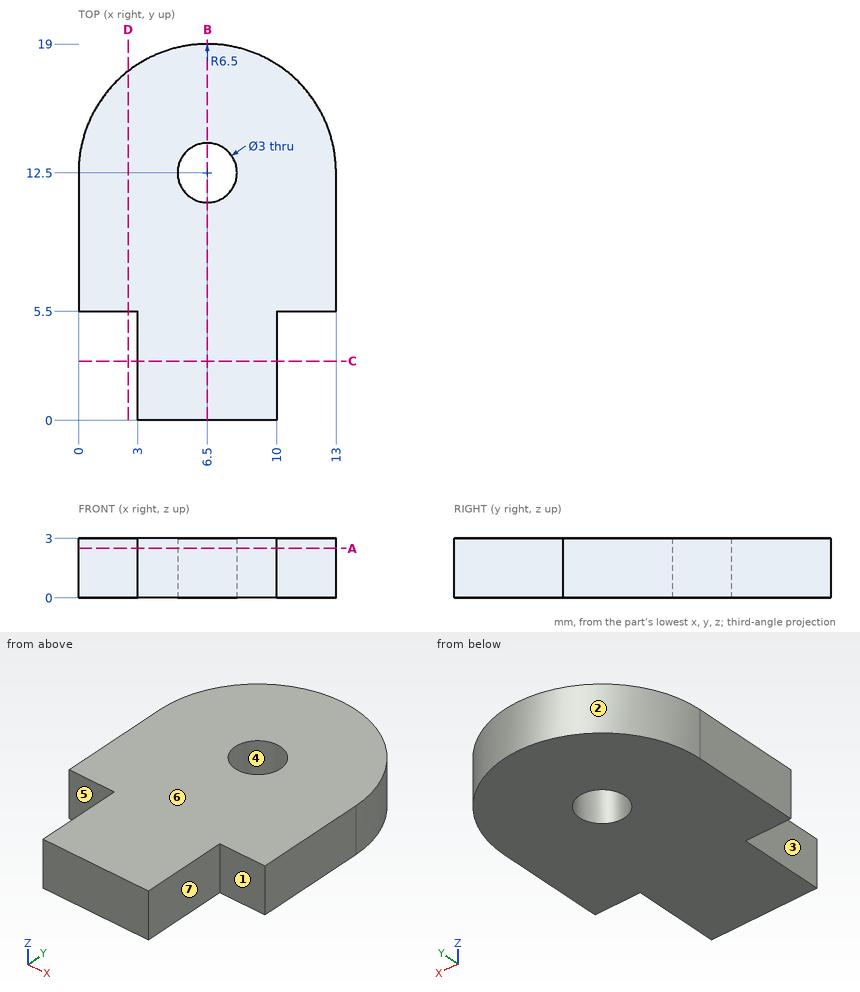
Check sheet for the drawn part. Datum: minimum x, y, z corner. Units: mm. A direction names the side the tool comes from. Round coordinates to 2 decimals unless told otherwise and drop trailing zeros. Loops run counter-clockwise (first coordinate to the right, second up) from the corner with the lowest first, then second, coordinate; pieces in that order, holes last. Notation, with made-up numbers: M 69.5,11 L 127.5,11 A37 ccw 127.5,49 Z; hole C -3.5,51.25 d10. An arc over 180 degrees is marked long. One line per question, with ' | ' between items. Start each with the question number.
Item 1: Release check for a two-part mould opening along Y. For the marked faces 1, 2, 3 and 4 record: released by +Y, released by -Y, zero draft, split by the parting line, or undercut.
Item 2: Set-up check for the marked faces 5, 6 and 7: record each of +Z, -Z, +X, -X, +Y, -Y from which the full face is reachable in a straight line by a thin tool's end or side.
Item 3: Section check A-A (z = 2.5). Record the boundary of the cut face in (x, y).
Item 4: Scan lines: probe 1 along Y at (x, z) = (6.5, 1.4); probe 2 along X at (y, z) = (4.5, 0.9); probe 3 along Y at (x, z) = (7, 2.55). Record each from-to range of solid material in increasing order.
Item 5: Section check C-C (y = 3). Record the boundary of the cut face in (x, z).
Item 6: Section check B-B (x = 6.5). Record the boundary of the cut face in (y, z).
Item 7: Gauge pin test, flat ends, axial feed: pin 1 Ø0.9 at (x, z) = (12, 2) entering from -Y; pin 2 Ø1.5 at (y, z) = (2, 1.5) entering from +X. Record the tip position at first contact, or that the pin passes through.
Item 8: Section check D-D (x = 2.5). Record the boundary of the cut face in (y, z), and give its area (3 significant figures).
Worked out:
1) face 1: released by -Y | face 2: released by +Y | face 3: zero draft | face 4: undercut
2) face 5: +Z, -Z, -X, -Y | face 6: +Z, +X, -X, +Y, -Y | face 7: +Z, -Z, +X, -Y
3) outline: M 0,5.5 L 3,5.5 L 3,0 L 10,0 L 10,5.5 L 13,5.5 L 13,12.5 A6.5 ccw 0,12.5 Z; hole C 6.5,12.5 d3
4) probe 1: 0 to 11, 14 to 19 | probe 2: 3 to 10 | probe 3: 0 to 11.09, 13.91 to 18.98
5) outline: M 3,0 L 10,0 L 10,3 L 3,3 Z
6) outline: M 0,0 L 11,0 L 11,3 L 0,3 Z; M 14,0 L 19,0 L 19,3 L 14,3 Z
7) pin 1: y = 5.5 | pin 2: x = 10
8) outline: M 5.5,0 L 17.62,0 L 17.62,3 L 5.5,3 Z | area: 36.4 mm^2
